CAD build for the part. Positions are in the model's coordinates, mm. A direction names the side the tool comes from. Round coordinates to 2 decimals unless told otherwise and drop trailing zeros. Loops run counter-clockwise (first coordinate to the right, second up) from the corner with the lowest first, then second, coordinate; pieces in that order, holes last.
```python
from build123d import *

# Parameters (mm, degrees)
SKETCH1_R           = 20
BOSS_EXTRUDE1_DEPTH = 500
BOSS_EXTRUDE2_DEPTH = 15
SKETCH4_R           = 10
BOSS_EXTRUDE3_DEPTH = 30


with BuildPart() as part:
    # Sketch1 → Boss-Extrude1 (new body)
    with BuildSketch(Plane.XY):
        Circle(SKETCH1_R)
    extrude(amount=BOSS_EXTRUDE1_DEPTH)

    # Sketch2 → Boss-Extrude2 (add, symmetric)
    with BuildSketch(Plane(origin=(0, 0, 0), x_dir=(1, 0, 0), z_dir=(0, 1, 0))):
        Polygon((-25, 40), (-15, 65), (15, 65), (25, 40), (25, 0), (-25, 0), align=None)
    extrude(amount=BOSS_EXTRUDE2_DEPTH, both=True)

    # Sketch4 → Boss-Extrude3 (add, symmetric)
    with BuildSketch(Plane(origin=(0, 0, 0), x_dir=(1, 0, 0), z_dir=(0, 1, 0))):
        with Locations(Location((0, 40, 0), (0, 0, 90))):
            Circle(SKETCH4_R)
    extrude(amount=BOSS_EXTRUDE3_DEPTH, both=True)


solid = part.part
```
Item 1: Cut at A-A, the plane y = 0. Give the cut face in (x, z).
Answers follow:
outline: (-25, -40) - (-15, -65) - (15, -65) - (25, -40) - (25, 0) - (20, 0) - (20, 500) - (-20, 500) - (-20, 0) - (-25, 0) - close
Item 2: 3-axis set-ups, long thin cutter, end or side, ignore diameter. For faces 1 (the flat face through (22, 0, 0)), 2 (the cylindrical face through (0, -22, -30)), 3 (the flat face through (0, 15, -26)), 4 (the cylindrical face through (-4.336, -19.524, 246.5)): which of +Z, -Z, +X, -X, +Y, -Y reach the whole face in a straight line?
Answers follow:
face 1: +Z, +X
face 2: -Y
face 3: +Y
face 4: +Z
Item 3: Cut at B-B, the plane z = 168. Give the cut face in (x, y), plus the area to 3 significant figures.
Answers follow:
outline: circle Ø40 at (0, 0)
area: 1,260 mm2
Item 4: Probe line 1 (Y direction, x = 15, z = 23.5); line 2 (Y direction, x = -2, z = 383); line 3 (X direction, y = -1.5, z = 70.5). List the from-to ranges inside material, lowest first.
Answers follow:
line 1: y = -13.23 to 13.23
line 2: y = -19.9 to 19.9
line 3: x = -19.94 to 19.94
Item 5: Flat gauge pins, fed straight in: P1, Ø6, axis at x = -17, z = 417.5, coming from the +Y side; P2, Ø12, axis at x = 19, z = 305, coming from the +Y side; P3, Ø4, axis at y = 18.5, z = 186, coming from the -X side. Where does each tip first touch, or does it go through?
Answers follow:
P1: stops at y = 14.28
P2: stops at y = 15.2
P3: stops at x = -11.3
Item 6: Two-plate mould, pull along Z, no slides. Class faces 5 (the flat face through (-25, 0, -20)), 6 (the flat face through (0, -15, -26)), 7 (the flat face through (0, 0, -65)): released by +Z, released by -Z, zero draft, split by the parting line, or undercut.
Answers follow:
face 5: zero draft
face 6: undercut
face 7: released by -Z
